Source: CAD feature listing. Evaluate the final solid. Frame: model axes, mm. A direction names the side the tool comes from. Round coordinates to 2 decimals unless told otherwise and drop trailing zeros. Order: outer loops, then holes, each group sorted by start corner. A loop starts at its lowest first (then second) coordinate and runs counter-clockwise, first axis right, second up. Notation, with made-up numbers: (-35, -27.5) -> (8, -27.5) arc R13 cw to (8, -5.5) -> close; hole circle Ø1 at (61.5, -38.75). An arc over 180 degrees is marked (long way). Answer as CSV lines item,"result". Start each with the question number.
(1) Line query: line 1 along X through (y, z) = (-20.75, 3.15); line 2 along X through (y, z) = (-20.75, 1.45); line 3 along Y through (x, z) = (-16.5, 3.8). Output: solid intervals per line, ascending. Write a range as from..to.
(2) Section query B-B (x = -21.5). Output: boundary loops of the cut face in (y, z), plus the area to 3 significant figures.
(3) Pull-direction query (Y, two-part tool) for faces 1 (the flat face through (-8.5, 0.4, 5)), 2 (the flat face through (0, 0, 2)), 3 (the flat face through (-18, -29.75, 2)); classes: +Y half, -Y half, draft (parallel to the pull), parting line (faces both ways), or undercut.
(4) Section query D-D (y = 15.5). Output: boundary loops of the cut face in (x, z) (3 decimals), plus the area to 3 significant figures.
(5) Contact query for flat-ended pins moving along their axis: P1, Ø1.2, axis at x = -18, z = 1, coming from the +Y side; P2, Ø2.5, axis at y = -3.5, z = 2.5, coming from the -X side (3 decimals); P3, Ø2.5, axis at y = -36, z = 2, coming from the -X side; P4, Ø2.5, axis at x = -24.56, y = -20.75, coming from the +Z side. Output: stop coordinate, or through.
(6) Set-up query: faces 4 (the flat face through (-4, -26.75, 2)), 5 (the flat face through (-18, 29.75, 2)), 6 (the conical face through (-10.376, -29.627, 1.82)). Return all of +Z, -Z, +X, -X, +Y, -Y with unobstructed straight access to the full face (end or side cutting, diameter ignored); none if empty.
(7) Section query A-A (y = -20.75). Output: boundary loops of the cut face in (x, z) (1 decimal), plus the area to 3 significant figures.
(8) Section query C-C (z = 4.15). Count the separate pieces of the cut face and the enclosed holes in it, plus the area to 3 significant figures.
Autodesk Inventor part; units mm, degrees
ref_plane "YZ Plane" through (0, 0, 0) normal (1, 0, 0) x (0, 1, 0)
ref_plane "XZ Plane" through (0, 0, 0) normal (0, 1, 0) x (-1, 0, 0)
ref_plane "XY Plane" through (0, 0, 0) normal (0, 0, 1) x (1, 0, 0)
sketch "Náčrt1" plane through (0, 0, 0) normal (0, 0, 1) x (1, 0, 0)
  line L0 (0, 0) -> (0, 26.75)
  line L1 (0, 26.75) -> (-30, 26.75)
  line L2 (-30, 26.75) -> (-30, 14.75)
  line L3 (-30, 14.75) -> (-8.875, 14.75)
  line L4 (-8.875, 14.75) -> (-8.875, 0)
  line L5 (-8.875, 0) -> (0, 0)
  circle A0 centre (-24.5625, 20.75) radius 1.5
  circle A1 centre (-4.4375, 20.75) radius 1.5
  line L6 (-19.125, 26.75) -> (-19.125, 14.75) construction
  dimension "d0" = 30
  dimension "d1" = 26.75
  dimension "d3" = 12
  dimension "d4" = 8.875
  dimension "d5" = 3
  dimension "d6" = 3
  dimension "d7" = 6
  dimension "d9" = 10.875
  dimension "d10" = 5.4375
  dimension "d11" = 4.4375
extrude "Vysunutí1" add sketch "Náčrt1" along normal blind 5
sketch "Náčrt2" plane through (-30, 26.75, 0) normal (0, 1, 0) x (1, 0, 0)
  circle A0 centre (16, 3.12) radius 6
  line L0 (30, 0) -> (0, 0)
  line L1 (21.125, 0) -> (21.125, -5)
  line L2 (30, -5) -> (0, -5)
  line L3 (10.875, -5) -> (10.875, 0)
  circle A1 centre (16, 3.12) radius 9
  point P0 (24.4419, 0)
  point P1 (7.5581, 0)
  dimension "d1" = 26.75
  dimension "d14" = 12
  dimension "d15" = 10.25
  dimension "d20" = 18
extrude "Vysunutí2" add sketch "Náčrt2" along normal blind 3 contours L3 A1 L0 | A0 L1 A1 L2 L3 | L0 A1 L1 | L2 A1
extrude "Vysunutí3" cut sketch "Náčrt2" against normal through all contours L0 A0 picked at (15.3305, -1.5618)
sketch "Náčrt3" plane through (0, 0, 5) normal (0, 0, 1) x (1, 0, 0)
  line L0 (-22.4419, 26.75) -> (-17.8815, 26.75)
  line L1 (0, 26.75) -> (-10.1185, 26.75)
  arc A0 (-17.8815, 26.75) -> (-10.1185, 26.75) centre (-14, 44.3265) ccw
  line L2 (-10.1185, 26.75) -> (-17.8815, 26.75)
  point P0 (0, 0)
  dimension "d21" = 18
revolve "Rotace1" add sketch "Náčrt3" angle 360 about axis through (-10.1185, 26.75, 5) along (-1, 0, 0)
sketch "Náčrt4" plane through (-30, 29.75, 0) normal (0, 1, 0) x (1, 0, 0)
  line L0 (21.125, 0) -> (21.125, -2.88)
  line L1 (21.125, 0) -> (21.125, -5)
  arc A0 (10.875, 0) -> (21.125, 0) centre (16, 3.12) ccw
  line L2 (10.875, -2.88) -> (10.875, 0)
  line L3 (21.125, -2.88) -> (10.875, -2.88)
  arc A1 (7.5581, 0) -> (24.4419, 0) centre (16, 3.12) ccw
  line L4 (24.4419, 0) -> (21.125, 0)
  line L5 (10.875, 0) -> (7.5581, 0)
  point P0 (30, 0)
extrude "Vysunutí4" add sketch "Náčrt4" along normal blind 9.25 contours L4 A1 L1 L0 | L1 A1 L5 L2 L3
chamfer "Zkosení1" distance 0.25 angle 45 2 edges at (-16.9394, 29.75, 2.1107) (-11.0606, 29.75, 2.1107)
mirror "Zrcadlit1" about plane through (-8.875, 0, 0) normal (0, -1, 0)
properties part number "joný=gej"
Answer block:
1,line 1,"-30..-26.06, -23.06..-5.94, -2.94..0"
1,line 2,"-30..-26.06, -23.06..-17.89, -10.11..-5.94, -2.94..0"
1,line 3,"-39..-14.75, 14.75..39"
2,outline,"(-39, 0) -> (-14.75, 0) -> (-14.75, 5) -> (-26.75, 5) -> (-26.75, 1.85) -> (-39, 1.85) -> close; (14.75, 0) -> (39, 0) -> (39, 1.85) -> (26.75, 1.85) -> (26.75, 5) -> (14.75, 5) -> close"
2,area,"165 mm2"
3,face 1,"undercut"
3,face 2,"draft"
3,face 3,"-Y half"
4,outline,"(-30, 0) -> (-19.125, 0) arc R6 cw to (-8.875, 0) -> (0, 0) -> (0, 5) -> (-30, 5) -> close"
4,area,"129 mm2"
5,P1,"y = 29.75"
5,P2,"x = -8.875"
5,P3,"x = -22.13"
5,P4,"through"
6,face 4,"+Z, +X, -Y"
6,face 5,"-Z, +Y"
6,face 6,"-Z, -Y"
7,outline,"(-30, 0) -> (-26.1, 0) -> (-26.1, 5) -> (-30, 5) -> close; (-23.1, 0) -> (-19.1, 0) arc R6 cw to (-8.9, 0) -> (-5.9, 0) -> (-5.9, 5) -> (-23.1, 5) -> close; (-2.9, 0) -> (0, 0) -> (0, 5) -> (-2.9, 5) -> close"
7,area,"99.1 mm2"
8,separate pieces,"1"
8,enclosed holes,"4"
8,area,"1,210 mm2"
